Autodesk Inventor part; units mm, degrees
ref_plane "YZ Plane" through (0, 0, 0) normal (1, 0, 0) x (0, 1, 0)
ref_plane "XZ Plane" through (0, 0, 0) normal (0, 1, 0) x (-1, 0, 0)
ref_plane "XY Plane" through (0, 0, 0) normal (0, 0, 1) x (1, 0, 0)
sketch "Sketch1" plane through (0, 0, 0) normal (0, 1, 0) x (-1, 0, 0)
  circle A0 centre (0, 0) radius 84.75
  dimension "d0" = 169.5
extrude "Extrusion1" add sketch "Sketch1" along normal blind 15
sketch "Sketch2" plane through (0, 0, 0) normal (0, -1, 0) x (1, 0, 0)
  circle A0 centre (0, 0) radius 76
  circle A1 centre (0, 76) radius 4
  circle A2 centre (0, -76) radius 4
  circle A3 centre (0, 76) radius 2.25
  circle A4 centre (0, -76) radius 2.25
  dimension "d3" = 152
  dimension "d4" = 8
  dimension "d5" = 8
  dimension "d6" = 4.5
  dimension "d7" = 4.5
extrude "Extrusion2" cut sketch "Sketch2" against normal through all contours A3 A0 | A0 A3 | A4 A0 | A0 A4
extrude "Extrusion3" cut sketch "Sketch2" against normal blind 12 contours A1 A0 A3 | A0 A3 A1 | A2 A0 A4 | A0 A4 A2 | A3 A0 | A0 A3 | A4 A0 | A0 A4
sketch "Sketch3" plane through (0, 15, 0) normal (0, 1, 0) x (1, 0, 0)
  circle A0 centre (0, 0) radius 84.75
hole "Hole1" at (0, 15, 0) direction (0, -1, 0) diameter 10.106 depth 12 countersink diameter 11.2 countersink angle 90
sketch "Sketch4" plane through (0, 15, 0) normal (0, 1, 0) x (1, 0, 0)
  circle A0 centre (0, 0) radius 5.053
  circle A1 centre (0, 0) radius 55
  line L0 (-55, -55) -> (55, -55)
  line L1 (55, -55) -> (55, 55)
  line L2 (55, 55) -> (-55, 55)
  line L3 (-55, 55) -> (-55, -55)
  line L4 (-55, -55) -> (55, 55) construction
  line L5 (55, -55) -> (-55, 55) construction
  circle A2 centre (-38.8909, -38.8909) radius 4
  circle A3 centre (-38.8909, 38.8909) radius 4
  circle A4 centre (38.8909, -38.8909) radius 4
  circle A5 centre (38.8909, 38.8909) radius 4
  dimension "d19" = 110
  dimension "d20" = 8
  dimension "d21" = 8
  dimension "d22" = 8
  dimension "d23" = 8
hole "Hole2" at (-38.8909, 15, 38.8909) at (-38.8909, 15, -38.8909) at (38.8909, 15, -38.8909) at (38.8909, 15, 38.8909) direction (0, -1, 0) diameter 6.647 depth 12
properties part number "substrate plate"
Check sheet for the modelled part. Datum: model origin and axes. Units: mm. A direction names the side the tool comes from. Round coordinates to 2 decimals unless told otherwise and drop trailing zeros. Loops run counter-clockwise (first coordinate to the right, second up) from the corner with the lowest first, then second, coordinate; pieces in that order, holes last.
1. Set-up check for faces 1 (the flat face through (-39, 3, 39)), 2 (the flat face through (2, 12, -78)), 3 (the cylindrical face through (-0.488, 13.479, -78.196)): record each of +Z, -Z, +X, -X, +Y, -Y from which the full face is reachable in a straight line by a thin tool's end or side.
2. Mould release check, pull along X, two halves, no side actions. Record for faces 4 (the flat face through (1, 0, 1)), 5 (the flat face through (-39, 3, -39)), 6 (the cylindrical face through (18.372, 7.395, 82.735)): released by +X, released by -X, zero draft, split by the parting line, or undercut.
3. Sectioned sample at D-D on z = 76. Record the boundary of the cut face in (x, y), and give its area (3 significant figures).
4. Gauge pin test, flat ends, axial feed: pin 1 Ø2 at (y, z) = (8, -18.5) entering from -X; pin 2 Ø4 at (x, y) = (39.5, 9) entering from -Z; pin 3 Ø3.5 at (x, z) = (40, 38) entering from +Y. Record the tip position at first contact, or that the pin passes through.
5. Scan lines: probe 1 along Z at (x, y) = (0, 8.75); probe 2 along X at (y, z) = (10.75, 0.5); probe 3 along Z at (x, y) = (-1, 5.25). Record each from-to range of solid material in increasing order.
6. Sectioned sample at A-A on x = 0. Record the boundary of the cut face in (y, z).
7. Sectioned sample at C-C on y = 7. Record the boundary of the cut face in (x, z), and give its area (3 significant figures).
8. Sectioned sample at B-B on z = 0. Record the boundary of the cut face in (x, y), and give its area (3 significant figures).
Recorded:
1. face 1: +Y
1. face 2: -Y
1. face 3: +Y, -Y
2. face 4: zero draft
2. face 5: undercut
2. face 6: split by the parting line
3. outline: (-37.5, 0) - (-4, 0) - (-4, 12) - (-2.25, 12) - (-2.25, 15) - (-37.5, 15) - close; (2.25, 12) - (4, 12) - (4, 0) - (37.5, 0) - (37.5, 15) - (2.25, 15) - close
3. area: 1,020 mm2
4. pin 1: stops at x = -82.92
4. pin 2: stops at z = -76
4. pin 3: stops at y = 3
5. probe 1: z = -84.75 to -80, -72 to -5.05, 5.05 to 72, 80 to 84.75
5. probe 2: x = -84.75 to -5.03, 5.03 to 84.75
5. probe 3: z = -84.74 to -79.87, -72.13 to -4.95, 4.95 to 72.13, 79.87 to 84.74
6. outline: (0, -84.75) - (15, -84.75) - (15, -78.25) - (12, -78.25) - (12, -80) - (0, -80) - close; (0, -72) - (12, -72) - (12, -73.75) - (15, -73.75) - (15, -5.6) - (14.45, -5.05) - (3, -5.05) - (3, 5.05) - (14.45, 5.05) - (15, 5.6) - (15, 73.75) - (12, 73.75) - (12, 72) - (0, 72) - close; (0, 80) - (12, 80) - (12, 78.25) - (15, 78.25) - (15, 84.75) - (0, 84.75) - close
7. outline: circle Ø169.5 at (0, 0); hole circle Ø6.65 at (-38.89, -38.89); hole circle Ø6.65 at (-38.89, 38.89); hole circle Ø10.11 at (0, 0); hole circle Ø8 at (0, -76); hole circle Ø8 at (0, 76); hole circle Ø6.65 at (38.89, -38.89); hole circle Ø6.65 at (38.89, 38.89)
7. area: 22,200 mm2
8. outline: (-84.75, 0) - (84.75, 0) - (84.75, 15) - (5.6, 15) - (5.05, 14.45) - (5.05, 3) - (-5.05, 3) - (-5.05, 14.45) - (-5.6, 15) - (-84.75, 15) - close
8. area: 2,420 mm2
